Design review of the part built by this model. Coordinates are the model's own, in mm. A direction names the side the tool comes from. Give positions to 0.01 mm unless a question says otherwise; leave off trailing zeros. Loops run counter-clockwise (first coordinate to the right, second up) from the corner with the lowest first, then second, coordinate; pieces in that order, holes last. Notation, with made-up numbers: (22, 34) -> (77, 34) arc R17 cw to (77, 57) -> close; hole circle Ø5 at (77, 16). An arc over 180 degrees is marked (long way). Use a Markdown table: item, result. Add a question column.
1. Draft analysis for pull direction Y (two halves, no side actions). For faces 5 (the flat face through (36, 0, 3)), 6 (the flat face through (-56, -42.5, 3)), 7 (the flat face through (30.702, 30.175, 2.958)), state which applies: pulls with the +Y half, pulls with the -Y half, needs draft (parallel to the pull), parting line crosses it, or undercut.
2. For faces 1 (the flat face through (-1, 12.5, 3)), 2 (the flat face through (-30.179, 29.825, 2.958)), 3 (the flat face through (-30.702, -30.175, 2.958)), 4 (the flat face through (-51.854, -25.079, 2.958)), list the 3-axis set-ups (+Z, -Z, +X, -X, +Y, -Y) from which the entire face can be reached by the end or side of a thin tool; tool diameter is ignored.
3. Add section D-D (y = -1.5). State the section outline as (x, z) points, and give its area (3 significant figures).
4. Add section A-A (z = 2.9). State the section outline as (x, y) points, and give its area (3 significant figures).
5. For pin 1 Ø1 at (x, z) = (-30.5, 4.5) entering from +Y; pin 2 Ø1.5 at (y, z) = (-5.5, 4) entering from +X; pin 3 Ø0.5 at (x, z) = (-40.5, 2) entering from +Y, all flat-tipped, find the tip position at first contact; note any pin that passes through.
6. To check wall thickness, follow line 1 (X direction, y = 0.5, z = 4.15); line 2 (Y direction, x = 8, z = 3.5); line 3 (Y direction, x = -4, z = 0.35). State the ranges of each line that lie inside material, in increasing order.
7. Add section B-B (x = 6). State the section outline as (y, z) points, and give its area (3 significant figures).
8. Add section C-C (y = -27.5). State the section outline as (x, z) points.
```python
from build123d import *

# Parameters (mm, degrees)
F0_W     = 72
F0_H     = 25
F1_DEPTH = 6
F2_DEPTH = 1


with BuildPart() as f1:
    # F0 (on Top) → F1 (new body)
    with BuildSketch(Plane.XY):
        Polygon((-49.116927, 42.5), (-63.5, 42.5), (-63.5, 32.873533), (-40.530132, 17.5), (-41, 17.5), (-41, -17.5), (-40.530132, -17.5), (-63.5, -32.873533), (-63.5, -42.5), (-49.116927, -42.5), (-11.763985, -17.5), (11.763985, -17.5), (49.116927, -42.5), (63.5, -42.5), (63.5, -32.873533), (40.530132, -17.5), (41, -17.5), (41, 17.5), (40.530132, 17.5), (63.5, 32.873533), (63.5, 42.5), (49.116927, 42.5), (11.763985, 17.5), (-11.763985, 17.5), align=None)
        Rectangle(F0_W, F0_H, mode=Mode.SUBTRACT)
    extrude(amount=F1_DEPTH)

    # F0 (on Top) → F2 (join)
    with BuildSketch(Plane.XY):
        Rectangle(F0_W, F0_H)
    extrude(amount=F2_DEPTH)


solid = f1.part
```
Taken from the geometry:
| question | item | result |
|---|---|---|
| 1 | face 5 | undercut |
| 1 | face 6 | pulls with the -Y half |
| 1 | face 7 | pulls with the +Y half |
| 2 | face 1 | +Z |
| 2 | face 2 | +Z, -Z, +Y |
| 2 | face 3 | +Z, -Z, -Y |
| 2 | face 4 | +Z, -Z, -X |
| 3 | outline | (-41, 0) -> (41, 0) -> (41, 6) -> (36, 6) -> (36, 1) -> (-36, 1) -> (-36, 6) -> (-41, 6) -> close |
| 3 | area | 132 mm^2 |
| 4 | outline | (-63.5, -42.5) -> (-49.12, -42.5) -> (-11.76, -17.5) -> (11.76, -17.5) -> (49.12, -42.5) -> (63.5, -42.5) -> (63.5, -32.87) -> (40.53, -17.5) -> (41, -17.5) -> (41, 17.5) -> (40.53, 17.5) -> (63.5, 32.87) -> (63.5, 42.5) -> (49.12, 42.5) -> (11.76, 17.5) -> (-11.76, 17.5) -> (-49.12, 42.5) -> (-63.5, 42.5) -> (-63.5, 32.87) -> (-40.53, 17.5) -> (-41, 17.5) -> (-41, -17.5) -> (-40.53, -17.5) -> (-63.5, -32.87) -> close; hole (-36, -12.5) -> (36, -12.5) -> (36, 12.5) -> (-36, 12.5) -> close |
| 4 | area | 3,670 mm^2 |
| 5 | pin 1 | stops at y = 30.37 |
| 5 | pin 2 | stops at x = 41 |
| 5 | pin 3 | stops at y = 36.9 |
| 6 | line 1 | x = -41 to -36, 36 to 41 |
| 6 | line 2 | y = -17.5 to -12.5, 12.5 to 17.5 |
| 6 | line 3 | y = -17.5 to 17.5 |
| 7 | outline | (-17.5, 0) -> (17.5, 0) -> (17.5, 6) -> (12.5, 6) -> (12.5, 1) -> (-12.5, 1) -> (-12.5, 6) -> (-17.5, 6) -> close |
| 7 | area | 85.0 mm^2 |
| 8 | outline | (-55.47, 0) -> (-26.71, 0) -> (-26.71, 6) -> (-55.47, 6) -> close; (26.71, 0) -> (55.47, 0) -> (55.47, 6) -> (26.71, 6) -> close |
